Check sheet for the modelled part. Datum: model origin and axes. Units: mm. Coordinates: 2 decimals unless noted, no trailing zeros. Write each loop counter-clockwise with the first axis right and the second up, starting at its lowest first coordinate (ties: lowest second). Pieces come first, ordered by that corner, then holes. Notation, with made-up numbers: (6.5, -0.5) -> (46.5, -0.5) arc R34 ccw to (46.5, 35.5) -> close; hole circle Ø9 at (-12.5, 25.5). An arc over 180 degrees is marked (long way). Put each result on its own line as item: value.
```python
from build123d import *

# Parameters (mm, degrees)
F0_R      = 5.08
F1_DEPTH  = 7.62
F2_R      = 1.27
F1_FACE_R = 3.81
F3_DEPTH  = 12.7


with BuildPart() as f1:
    # F0 (on Top) → F1 (new body)
    with BuildSketch(Plane.XY):
        Circle(F0_R)
    extrude(amount=F1_DEPTH)

    # F2
    f2_edges = [f1.edges().sort_by_distance(p)[0] for p in [
        (-5.08, 0, 7.62),
    ]]
    fillet(f2_edges, radius=F2_R)

    # F1_face (on face) → F3 (join)
    with BuildSketch(Plane.XY.offset(7.62)):
        Circle(F1_FACE_R)
    extrude(amount=F3_DEPTH)


solid = f1.part
```
Q1. Depth check by flat-ended pin: P1, Ø3, axis at y = 2, z = 16.5, coming from the -X side; P2, Ø3, axis at y = -2, z = 7.5, coming from the -X side; P3, Ø1.5, axis at y = 0.5, z = 18, coming from the +X side. Enter the tip coordinate at first touch or a pass-through.
Recorded:
P1: stops at x = -3.78
P2: stops at x = -4.99
P3: stops at x = 3.81
Q2. Cross-section at C-C (z = 5.5). Record the cut outline in (x, y).
Recorded:
outline: circle Ø10.16 at (0, 0)
Q3. Mould release check, pull along Y, two halves, no side actions. Record for faces 1 (the cylindrical face through (-0.83, -3.72, 13.88)), 2 (the flat face through (0, 0, 0)): released by +Y, released by -Y, zero draft, split by the parting line, or undercut.
Recorded:
face 1: split by the parting line
face 2: zero draft
Q4. Cross-section at A-A (y = 0). Record the cut outline in (x, z), plus the area to 3 significant figures.
Recorded:
outline: (-5.08, 0) -> (5.08, 0) -> (5.08, 6.35) arc R1.27 ccw to (3.81, 7.62) -> (3.81, 20.32) -> (-3.81, 20.32) -> (-3.81, 7.62) arc R1.27 ccw to (-5.08, 6.35) -> close
area: 174 mm2
Q5. Material ranges on line 1 along Y through (x, z) = (3.5, 3.5); line 2 along Z through (x, y) = (-3.5, -3); line 3 along X through (y, z) = (-0.25, 5), recorded low to high.
Recorded:
line 1: y = -3.68 to 3.68
line 2: z = 0 to 7.34
line 3: x = -5.07 to 5.07
